Verification items for the finished model (mm, model axes). Face numbers are marked on the shaded views. A direction names the side the tool comes from. Give positions to 0.01 mm unless a question says otherwise; leave off trailing zeros. Write each loop counter-clockwise with the first axis right and the second up, starting at its lowest first coordinate (ties: lowest second). Pieces come first, ordered by that corner, then holes. Notation, with made-up numbers: M -33,-34.5 L -28,-34.5 A27 ccw -28,-8.5 Z; hole C 33,65.5 d1. An arc over 180 degrees is marked long. Answer as a JSON object with one key per item and string values.
```python
from build123d import *

# Parameters (mm, degrees)
SKETCH1_R           = 21
BOSS_EXTRUDE1_DEPTH = 35
SKETCH2_R           = 8
BOSS_EXTRUDE2_DEPTH = 1
SKETCH3_R           = 2.5
BOSS_EXTRUDE3_DEPTH = 10
BOSS_EXTRUDE4_START = -10
SKETCH4_W           = 23
SKETCH4_H           = 14.139392284
BOSS_EXTRUDE4_DEPTH = 5
SKETCH6_R           = 1.25
CUT_EXTRUDE1_DEPTH  = 5


with BuildPart() as part:
    # Sketch1 → Boss-Extrude1 (new body)
    with BuildSketch(Plane.XY):
        Circle(SKETCH1_R)
    extrude(amount=BOSS_EXTRUDE1_DEPTH)

    # Sketch2 → Boss-Extrude2 (add)
    with BuildSketch(Plane.XY.offset(35)):
        Circle(SKETCH2_R)
    extrude(amount=BOSS_EXTRUDE2_DEPTH)

    # Sketch3 → Boss-Extrude3 (add)
    with BuildSketch(Plane.XY.offset(36)):
        Circle(SKETCH3_R)
    extrude(amount=BOSS_EXTRUDE3_DEPTH)

    # Sketch4 → Boss-Extrude4 (add)
    with BuildSketch(Plane(origin=(0, 0, 0), x_dir=(-1, 0, 0), z_dir=(0, 0, -1)).offset(BOSS_EXTRUDE4_START)):
        with Locations((0, 20.930303858)):
            Rectangle(SKETCH4_W, SKETCH4_H)
    extrude(amount=-BOSS_EXTRUDE4_DEPTH)

    # Sketch6 → Cut-Extrude1 (cut)
    with BuildSketch(Plane.XY.offset(35)):
        with Locations((0, -15)):
            Circle(SKETCH6_R)
        with Locations((-12.990381057, 7.5)):
            Circle(SKETCH6_R)
        with Locations((12.990381057, 7.5)):
            Circle(SKETCH6_R)
    extrude(amount=-CUT_EXTRUDE1_DEPTH, mode=Mode.SUBTRACT)


solid = part.part
```
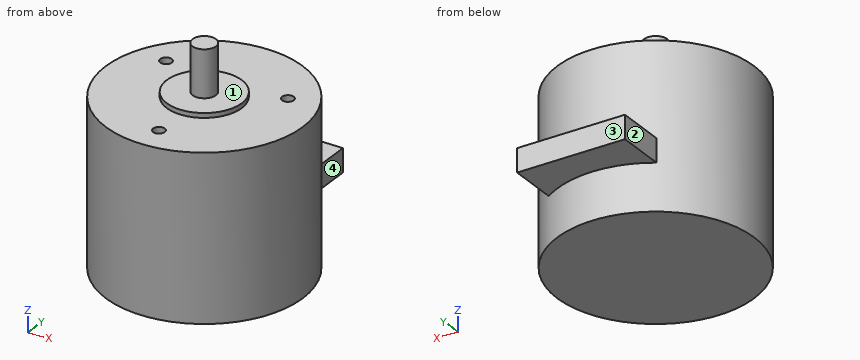
1) Access from +Z, -Z, +X, -X, +Y, -Y to the whole of each face (thin tool, end or side, straight path). Record for the marked faces 1, 2, 3 and 4.
Completed:
{"face 1": "+Z", "face 2": "+Z, -Z, -X, +Y", "face 3": "+Z, -Z, +X, -X, +Y", "face 4": "+Z, -Z, +X, +Y"}
2) Section check A-A on y = 0. Record the boundary of the cut face in (x, z), and give its area (3 significant figures).
Completed:
{"outline": "M -21,0 L 21,0 L 21,35 L 8,35 L 8,36 L 2.5,36 L 2.5,46 L -2.5,46 L -2.5,36 L -8,36 L -8,35 L -21,35 Z", "area": "1,540 mm2"}
3) Section check C-C on z = 42.5. Record the boundary of the cut face in (x, y), and give its area (3 significant figures).
Completed:
{"outline": "C 0,0 d5", "area": "19.6 mm2"}
4) Section check D-D on y = 25. Record the boundary of the cut face in (x, z), and give its area (3 significant figures).
Completed:
{"outline": "M -11.5,10 L 11.5,10 L 11.5,15 L -11.5,15 Z", "area": "115 mm2"}
5) Section check B-B on x = 0. Record the boundary of the cut face in (y, z), and give its area (3 significant figures).
Completed:
{"outline": "M -21,0 L 21,0 L 21,10 L 28,10 L 28,15 L 21,15 L 21,35 L 8,35 L 8,36 L 2.5,36 L 2.5,46 L -2.5,46 L -2.5,36 L -8,36 L -8,35 L -13.75,35 L -13.75,30 L -16.25,30 L -16.25,35 L -21,35 Z", "area": "1,560 mm2"}
6) Go/stop test with flat-tipped pins: pin 1 (3 mm diameter, centred on x = -13, y = 7.5, fed in from +Z); pin 2 (4 mm diameter, centred on x = -16, z = 26, fed in from -Y); pin 3 (4 mm diameter, centred on y = 25, z = 11.5, fed in from -X). Record where each tip stops, or that it passes through.
Completed:
{"pin 1": "stops at z = 35", "pin 2": "stops at y = -15.65", "pin 3": "stops at x = -11.5"}
7) Thickness scan on L1, parallel to Y at x = 0, z = 31.9; L2, parallel to Z at x = 1, y = -4; L3, parallel to Z at x = 17, y = 8.5. Record the ranges inside material, lowest first.
Completed:
{"L1": "y = -21 to -16.25, -13.75 to 21", "L2": "z = 0 to 36", "L3": "z = 0 to 35"}
